Geometry: final body of the model. Coordinates: model frame, mm. Give positions to 0.01 mm unless a question says otherwise; leave off trailing zeros. Write each loop counter-clockwise with the first axis right and the second up, starting at its lowest first coordinate (ties: lowest second). Pieces come first, ordered by that corner, then holes. Notation, with made-up numbers: (-12, 83) - (-2, 83) arc R4 ccw to (-2, 90) - close; hole circle Ø6 at (-20, 49.25). An arc over 180 degrees is marked (long way). One line per question, with ' | ' between items. Start each with the question number.
```python
from build123d import *

# Parameters (mm, degrees)
F0_W     = 88.9
F0_H     = 152.4
F1_DEPTH = 6.35
F2_R     = 5.08
F3_W     = 2.027904
F3_H     = 29.865486
F4_DEPTH = 5.08
F5_R     = 0.508


with BuildPart() as f1:
    # F0 (on Front) → F1 (new body, symmetric)
    with BuildSketch(Plane.XZ):
        Rectangle(F0_W, F0_H)
    extrude(amount=F1_DEPTH, both=True)

    # F2
    f2_edges = [f1.edges().sort_by_distance(p)[0] for p in [
        (0, -6.35, 76.2),
        (-44.45, -6.35, 0),
        (0, -6.35, -76.2),
        (44.45, -6.35, 0),
        (-44.45, 0, 76.2),
        (-44.45, 0, -76.2),
        (44.45, 0, -76.2),
        (44.45, 0, 76.2),
    ]]
    fillet(f2_edges, radius=F2_R)

    # F3 (on face) → F4 (cut)
    with BuildSketch(Plane.YZ.offset(44.45)):
        with Locations((3.185241, 9.586453)):
            Rectangle(F3_W, F3_H)
    extrude(amount=-F4_DEPTH, mode=Mode.SUBTRACT)

    # F5
    f5_edges = [f1.edges().sort_by_distance(p)[0] for p in [
        (39.37, 4.199193, 9.586453),
        (39.37, 2.171289, 9.586453),
        (39.37, 3.185241, -5.34629),
        (44.45, 3.185241, 24.519196),
    ]]
    fillet(f5_edges, radius=F5_R)


solid = f1.part
```
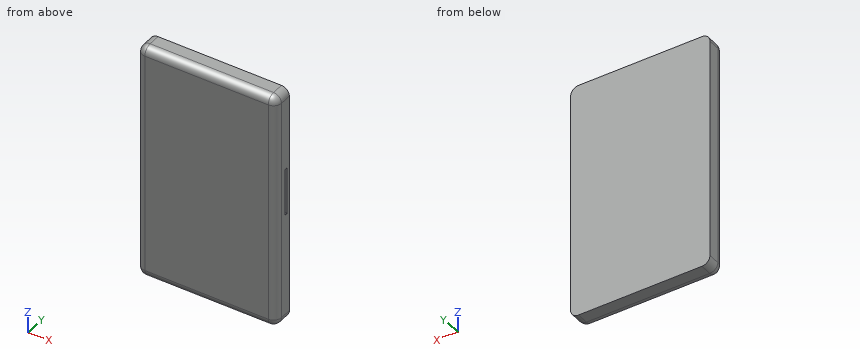
1) First-contact query: pin 1 Ø1 at (x, y) = (41.5, 3) entering from -Z; pin 2 Ø2 at (y, z) = (-4, 14) entering from +X; pin 3 Ø1.4 at (x, z) = (42, 5.5) entering from -Y. Flat tips, straight axial feed; report the tip coordinate or a pass-through.
2) Section B-B, the plane y = -3.75. Output: boundary loops of the cut face in (x, z), plus the area to 3 significant figures.
3) Line query: L1, parallel to X at y = 2.5, z = 16.5; L2, parallel to Z at x = 7, y = -1.75; L3, parallel to Z at x = 27.5, y = -4.25. Output: solid intervals per line, ascending.
4) Section A-A, the plane z = 9. Output: boundary loops of the cut face in (x, y), plus the area to 3 significant figures.
Answer key:
1) pin 1: z = -75.93 | pin 2: x = 44.15 | pin 3: y = -5.97
2) outline: (-43.8, -71.12) arc R4.43 ccw to (-39.37, -75.55) - (39.37, -75.55) arc R4.43 ccw to (43.8, -71.12) - (43.8, 71.12) arc R4.43 ccw to (39.37, 75.55) - (-39.37, 75.55) arc R4.43 ccw to (-43.8, 71.12) - close | area: 13,200 mm^2
3) L1: -44.45 to 39.4 | L2: -76.18 to 76.18 | L3: -75.23 to 75.23
4) outline: (-44.45, -1.27) arc R5.08 ccw to (-39.37, -6.35) - (39.37, -6.35) arc R5.08 ccw to (44.45, -1.27) - (44.45, 2.17) - (39.88, 2.17) arc R0.51 cw to (39.37, 2.68) - (39.37, 3.69) arc R0.51 cw to (39.88, 4.2) - (44.45, 4.2) - (44.45, 6.35) - (-44.45, 6.35) - close | area: 1,110 mm^2
